Read the model definition and answer for the solid it produces. Units are mm, in the model's axes. Give positions to 0.01 mm unless a question says otherwise; leave off trailing zeros. Order: outer loops, then holes, each group sorted by start corner. A loop starts at its lowest first (then second) coordinate and runs counter-clockwise, first axis right, second up. Notation, with made-up numbers: (89.25, -27.75) - (131.25, -27.75) arc R21 cw to (131.25, -18.75) - close; hole circle Ø10 at (22, -31.5). An arc over 180 degrees is marked (long way). One line per item, written item: value. Start each with the question number.
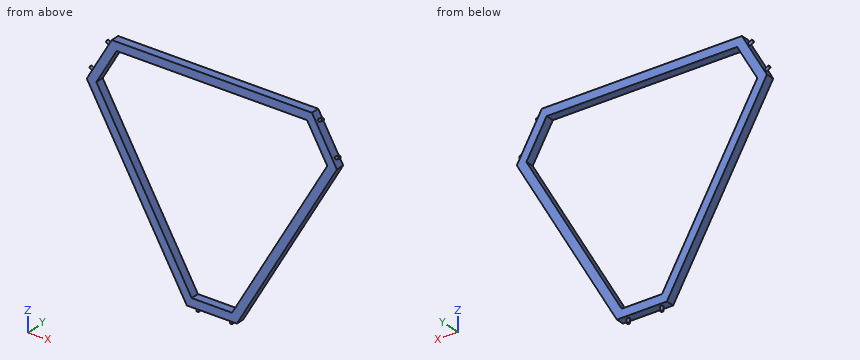
```python
from build123d import *

# Parameters (mm, degrees)
BOSS_EXTRUDE1_DEPTH = 50
SKETCH2_R           = 8
BOSS_EXTRUDE2_DEPTH = 25
CIRPATTERN1_COUNT   = 3


with BuildPart() as part:
    # Sketch1 → Boss-Extrude1 (new body)
    with BuildSketch(Plane(origin=(0, 0, 0), x_dir=(1, 0, 0), z_dir=(0, 1, 0))):
        Polygon((-600, -519.615242271), (600, -519.615242271), (750, -259.807621135), (150, 779.422863406), (-150, 779.422863406), (-750, -259.807621135), align=None)
        Polygon((-121.132486541, 729.422863406), (-692.264973081, -259.807621135), (-571.132486541, -469.615242271), (571.132486541, -469.615242271), (692.264973081, -259.807621135), (121.132486541, 729.422863406), align=None, mode=Mode.SUBTRACT)
    extrude(amount=BOSS_EXTRUDE1_DEPTH)

    # Sketch2 → Boss-Extrude2 (add)
    with BuildSketch(Plane(origin=(675, 0, 389.711431703), x_dir=(0.5000000000000172, 0, -0.8660254037844287), z_dir=(0.8660254037844287, 0, 0.5000000000000172))):
        with Locations(Location((-100, 25, 0), (0, 0, 180))):
            Circle(SKETCH2_R)
        with Locations(Location((100, 25, 0), (0, 0, 180))):
            Circle(SKETCH2_R)
    boss_extrude2 = extrude(amount=BOSS_EXTRUDE2_DEPTH)

    # CirPattern1: Boss-Extrude2 ×3 about axis
    cirpattern1_axis = Axis((0, 0, 0), (0, 1, 0))
    for i in range(1, CIRPATTERN1_COUNT):
        add(boss_extrude2.rotate(cirpattern1_axis, i * 360 / CIRPATTERN1_COUNT))


solid = part.part
```
1) Section B-B on x = 274.5 is taken. Write down the section's boundary in (y, z), plus the area to 3 significant figures.
2) Each of these flat-tipped pins is pushed along its axis until it touches: pin 1 (12 mm diameter, centred on x = -17.5, y = 38, fed in from -Z); pin 2 (25 mm diameter, centred on x = -279.5, y = 36, fed in from -Z); pin 3 (5 mm diameter, centred on x = -253, y = 44.5, fed in from -Z). Where does it stop, or does it pass through?
3) Find the intervals of material crossed by probe 1 along Z at (x, y) = (114, 11); probe 2 along X at (y, z) = (34.5, 260); probe 3 along Z at (x, y) = (-488.5, 37), in increasing order. Write a range as from..to.
4) Section A-A on y = 7.5 is taken. Write down the section's boundary in (x, z), plus the area to 3 significant figures.
5) Section C-C on z = 24 is taken. Write down the section's boundary in (x, y), plus the area to 3 significant figures.
Solved:
1. outline: (0, -563.78) - (50, -563.78) - (50, -463.78) - (0, -463.78) - close; (0, 469.62) - (50, 469.62) - (50, 519.62) - (0, 519.62) - close
1. area: 7,500 mm2
2. pin 1: stops at z = -779.42
2. pin 2: stops at z = -576.77
2. pin 3: stops at z = -605.35
3. probe 1: z = -779.42..-729.42, 469.62..519.62
3. probe 2: x = -749.89..-692.15, 692.15..749.89
3. probe 3: z = -193.12..-93.12, 469.62..519.62
4. outline: (-750, 259.81) - (-150, -779.42) - (150, -779.42) - (750, 259.81) - (600, 519.62) - (-600, 519.62) - close; hole (-692.26, 259.81) - (-121.13, -729.42) - (121.13, -729.42) - (692.26, 259.81) - (571.13, 469.62) - (-571.13, 469.62) - close
4. area: 216,000 mm2
5. outline: (-613.86, 0) - (-556.12, 0) - (-556.12, 50) - (-613.86, 50) - close; (556.12, 0) - (613.86, 0) - (613.86, 50) - (556.12, 50) - close
5. area: 5,770 mm2
